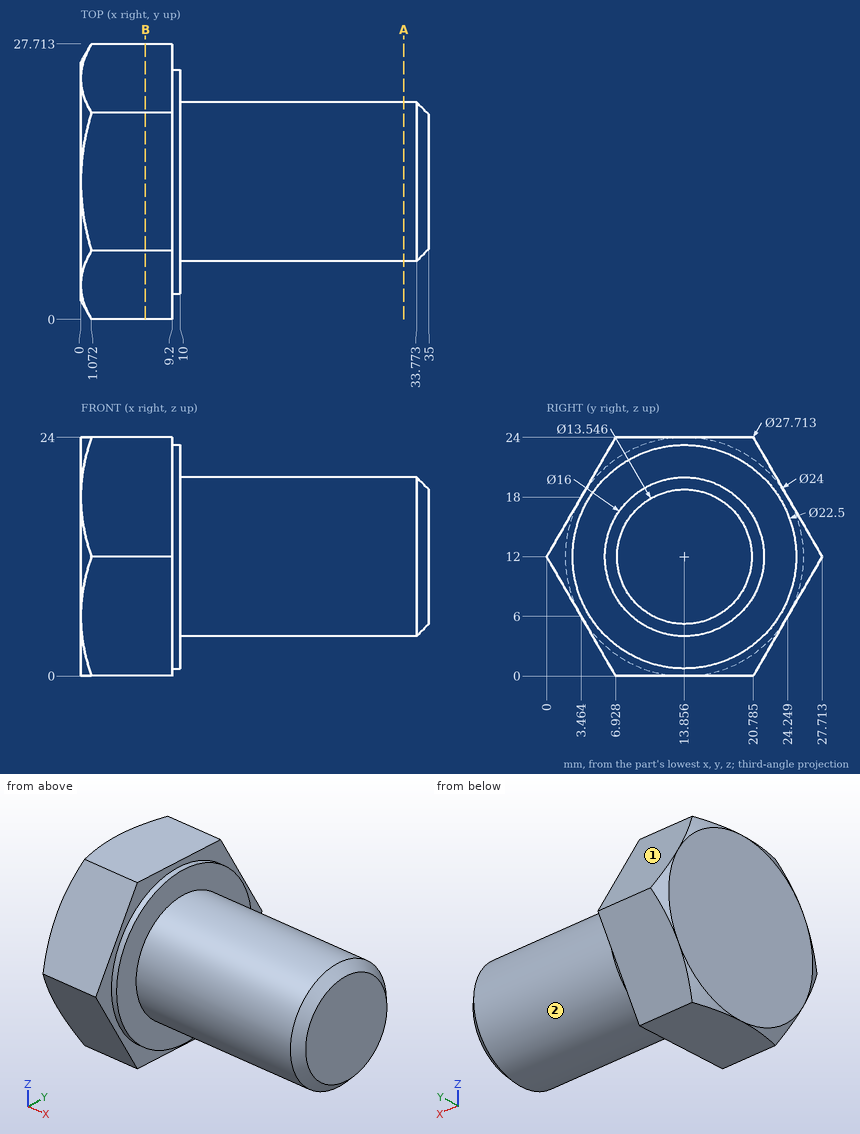
The figure shows three views and two pictorial views of one solid part (mm, origin at its lowest corner). Answer the questions. A direction names the side the tool comes from. Coordinates: 2 decimals unless noted, no trailing zeros. Write each loop counter-clockwise with the first axis right and the second up, starting at its lowest first coordinate (ties: lowest second). Pieces come first, ordered by that corner, then holes. Notation, with made-up numbers: (23.25, 44.25) -> (35.25, 44.25) arc R19 cw to (35.25, 65.25) -> close; hole circle Ø7 at (-2, 28.25). An arc over 180 degrees is marked (long way). Return JSON: item names as keys, results as strings.
(1) The part is cut by section A-A on x = 32.5. Give the vertices of the cut face in (y, z), then the cut area to 3 significant figures.
Answers below:
{"outline": "circle Ø16 at (13.86, 12)", "area": "201 mm^2"}
(2) Which of the six approach directions +Z, -Z, +X, -X, +Y, -Y give full straight-line access (tool end or side, diameter ignored) to the marked faces 1 and 2?
Answers below:
{"face 1": "+Z, +X, -X, +Y", "face 2": "+X"}
(3) The part is cut by section B-B on x = 6.5. Give the vertices of the cut face in (y, z) (1 decimal), then the cut area to 3 significant figures.
Answers below:
{"outline": "(0, 12) -> (6.9, 0) -> (20.8, 0) -> (27.7, 12) -> (20.8, 24) -> (6.9, 24) -> close", "area": "499 mm^2"}
(4) Consider line 1 along X through (y, z) = (7.25, 20); line 2 along Y through (x, z) = (19, 6.75); line 3 along Z through (x, y) = (8.5, 23.75) (1 decimal). Determine where each line is inside the solid, lowest interval first. Write a range as from..to.
Answers below:
{"line 1": "0..10", "line 2": "7.82..19.89", "line 3": "5.1..18.9"}
(5) Each of these flat-tipped pins is pushed along its axis until it touches: P1, Ø1.5, axis at x = 24.5, z = 6, coming from the +Y side; P2, Ø5, axis at x = 20, y = 15.5, coming from the +Z side; P3, Ø5, axis at x = 7.5, z = 15, coming from the +Y side (1 decimal); P4, Ø2, axis at y = 9, z = 17.5, coming from the +X side. Where does it stop, or does it pass through?
Answers below:
{"P1": "y = 19.89", "P2": "z = 20", "P3": "y = 27.4", "P4": "x = 35"}
